For this review, take the finished solid that the model builds, in its own axes (mm). Face numbers are marked on the shaded views. A direction names the side the tool comes from. Round coordinates to 2 decimals unless told otherwise and drop trailing zeros. Order: outer loops, then holes, each group sorted by start corner. A loop starts at its lowest first (then second) coordinate and runs counter-clockwise, first axis right, second up. Notation, with made-up numbers: (26, 69.25) -> (58, 69.25) arc R33 ccw to (58, 98.25) -> close; hole circle Ø2 at (-14, 60.25). An arc over 180 degrees is marked (long way). Use a Markdown table: item, result. Add a question column.
1) Consider section D-D (y = 3.5). State the section outline as (x, z) points, plus the area to 3 significant figures.
2) Draft analysis for pull direction X (two halves, no side actions). For the marked faces 1, 2, 3 and 4, state which applies: pulls with the +X half, pulls with the -X half, needs draft (parallel to the pull), parting line crosses it, or undercut.
3) Wall thickness on line 1 along Y through (x, z) = (3.5, 1.3); line 2 along X through (y, z) = (2.5, 2.5); line 3 along Z through (x, y) = (54.25, -1): over which ranges is each line inside the solid? List them lowest first. Write a range as [from, to].
4) Clearance check with flat-ended pins moving along their axes: P1, Ø1, axis at x = 86, y = 44.5, coming from the -Z side; P2, Ø12, axis at x = 65.5, y = 27.5, coming from the -Z side; P3, Ø3, axis at x = 56, z = 5.5, coming from the +Y side. State where each tip first meets the part, or that it passes through.
5) Consider section B-B (x = 3.5). State the section outline as (y, z) points.
6) Machinability: for the marked faces 5, 6, 7 and 8, which of the approach directions +Z, -Z, +X, -X, +Y, -Y give a long, thin tool a straight path to every point of the face, cutting with its end or side? Answer none if there is none.
7) Consider section C-C (z = 12.25). State the section outline as (x, y) points.
8) Consider section A-A (y = 52.5). State the section outline as (x, z) points, plus the area to 3 significant figures.
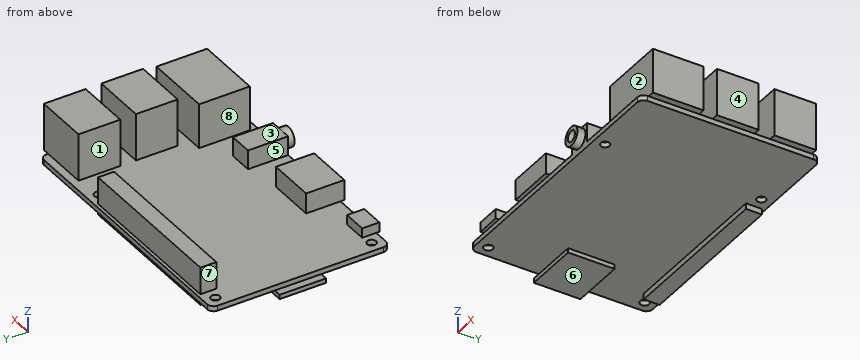
```python
from build123d import *

# Parameters (mm, degrees)
F0_R      = 1.4
F1_DEPTH  = 1.6
F2_W      = 15.1
F2_H      = 13.1
F2_W_2    = 2.1
F3_DEPTH  = 14.8
F2_W_3    = 19.1
F2_H_2    = 15.9
F4_DEPTH  = 14
F5_W      = 50.8
F5_H      = 5
F6_DEPTH  = 8.5
F7_DEPTH  = 3.4
F8_W      = 17
F8_H      = 14.6
F9_DEPTH  = 1.4
F10_W     = 7.5
F10_H     = 4.4
F10_H_2   = 1
F11_DEPTH = 3
F10_W_2   = 15
F10_H_3   = 10.8
F10_H_4   = 1.2
F12_DEPTH = 6.4
F10_H_5   = 12.6
F13_DEPTH = 6
F14_R     = 3
F14_R_2   = 1.75
F15_DEPTH = 2.5


with BuildPart() as f1:
    # F0 (on Top) → F1 (new body)
    with BuildSketch(Plane.XY):
        with BuildLine():
            ThreePointArc((0, 2), (0.585786, 0.585786), (2, 0))
            Line((2, 0), (83, 0))
            ThreePointArc((83, 0), (84.414214, 0.585786), (85, 2))
            Line((85, 2), (85, 54))
            ThreePointArc((85, 54), (84.414214, 55.414214), (83, 56))
            Line((83, 56), (2, 56))
            ThreePointArc((2, 56), (0.585786, 55.414214), (0, 54))
            Line((0, 54), (0, 2))
        make_face()
        with Locations((3.5, 3.5)):
            Circle(F0_R, mode=Mode.SUBTRACT)
        with Locations((61.5, 3.5)):
            Circle(F0_R, mode=Mode.SUBTRACT)
        with Locations((3.5, 52.5)):
            Circle(F0_R, mode=Mode.SUBTRACT)
        with Locations((61.5, 52.5)):
            Circle(F0_R, mode=Mode.SUBTRACT)
    extrude(amount=F1_DEPTH)

    # F2 (on face) → F3 (join)
    with BuildSketch(Plane.XY.offset(1.6)):
        with Locations((77.45, 46.95)):
            Rectangle(F2_W, F2_H)
        with Locations((86.05, 46.95)):
            Rectangle(F2_W_2, F2_H)
        with Locations((77.45, 28.95)):
            Rectangle(F2_W, F2_H)
        with Locations((86.05, 28.95)):
            Rectangle(F2_W_2, F2_H)
    extrude(amount=F3_DEPTH)

    # F2 (on face) → F4 (join)
    with BuildSketch(Plane.XY.offset(1.6)):
        with Locations((75.45, 10.25)):
            Rectangle(F2_W_3, F2_H_2)
        with Locations((86.05, 10.25)):
            Rectangle(F2_W_2, F2_H_2)
    extrude(amount=F4_DEPTH)

    # F5 (on face) → F6 (join)
    with BuildSketch(Plane.XY.offset(1.6)):
        with Locations((32.4, 52.5)):
            Rectangle(F5_W, F5_H)
    extrude(amount=F6_DEPTH)

    # F5 (on face) → F7 (join)
    with BuildSketch(Plane.XY.offset(1.6)):
        with Locations((32.4, 52.5)):
            Rectangle(F5_W, F5_H)
    extrude(amount=-F7_DEPTH)

    # F8 (on face) → F9 (join)
    with BuildSketch(Plane(origin=(0, 0, 0), x_dir=(1, 0, 0), z_dir=(0, 0, -1))):
        with Locations((6.1, -28.8)):
            Rectangle(F8_W, F8_H)
    extrude(amount=F9_DEPTH)

    # F10 (on face) → F11 (join)
    with BuildSketch(Plane.XY.offset(1.6)):
        with Locations((10.55, 2.2)):
            Rectangle(F10_W, F10_H)
        with Locations((10.55, -0.5)):
            Rectangle(F10_W, F10_H_2)
    extrude(amount=F11_DEPTH)

    # F10 (on face) → F12 (join)
    with BuildSketch(Plane.XY.offset(1.6)):
        with Locations((32, 5.4)):
            Rectangle(F10_W_2, F10_H_3)
        with Locations((32, -0.6)):
            Rectangle(F10_W_2, F10_H_4)
    extrude(amount=F12_DEPTH)

    # F10 (on face) → F13 (join)
    with BuildSketch(Plane.XY.offset(1.6)):
        with Locations((54.25, 6.3)):
            Rectangle(F10_W, F10_H_5)
    extrude(amount=F13_DEPTH)

    # F14 (on face) → F15 (join)
    with BuildSketch(Plane.XZ):
        with Locations((54.25, 4.6)):
            Circle(F14_R)
        with Locations((54.25, 4.6)):
            Circle(F14_R_2, mode=Mode.SUBTRACT)
    extrude(amount=F15_DEPTH)


solid = f1.part
```
Results list:
| question | item | result |
|---|---|---|
| 1 | outline | (0, 0) -> (2.1, 0) -> (2.1, 1.6) -> (0, 1.6) -> close; (4.9, 0) -> (60.1, 0) -> (60.1, 1.6) -> (58, 1.6) -> (58, 7.6) -> (50.5, 7.6) -> (50.5, 1.6) -> (39.5, 1.6) -> (39.5, 8) -> (24.5, 8) -> (24.5, 1.6) -> (14.3, 1.6) -> (14.3, 4.6) -> (6.8, 4.6) -> (6.8, 1.6) -> (4.9, 1.6) -> close; (62.9, 0) -> (85, 0) -> (85, 1.6) -> (87.1, 1.6) -> (87.1, 15.6) -> (65.9, 15.6) -> (65.9, 1.6) -> (62.9, 1.6) -> close |
| 1 | area | 587 mm2 |
| 2 | face 1 | undercut |
| 2 | face 2 | needs draft |
| 2 | face 3 | undercut |
| 2 | face 4 | pulls with the +X half |
| 3 | line 1 | [0, 2.1], [4.9, 51.1], [53.9, 56] |
| 3 | line 2 | [6.8, 14.3], [24.5, 39.5], [50.5, 58], [65.9, 87.1] |
| 3 | line 3 | [1.6, 2.85], [6.35, 7.6] |
| 4 | P1 | z = 1.6 |
| 4 | P2 | z = 0 |
| 4 | P3 | y = 55 |
| 5 | outline | (0, 0) -> (2.1, 0) -> (2.1, 1.6) -> (0, 1.6) -> close; (4.9, 0) -> (21.5, 0) -> (21.5, -1.4) -> (36.1, -1.4) -> (36.1, 0) -> (51.1, 0) -> (51.1, 1.6) -> (4.9, 1.6) -> close; (53.9, 0) -> (56, 0) -> (56, 1.6) -> (53.9, 1.6) -> close |
| 6 | face 5 | +Z, -Y |
| 6 | face 6 | -Z, +X, -X, -Y |
| 6 | face 7 | +Z, -X, +Y |
| 6 | face 8 | +Z, +Y, -Y |
| 7 | outline | (65.9, 2.3) -> (87.1, 2.3) -> (87.1, 18.2) -> (65.9, 18.2) -> close; (69.9, 22.4) -> (87.1, 22.4) -> (87.1, 35.5) -> (69.9, 35.5) -> close; (69.9, 40.4) -> (87.1, 40.4) -> (87.1, 53.5) -> (69.9, 53.5) -> close |
| 8 | outline | (0, 0) -> (2.1, 0) -> (2.1, 1.6) -> (0, 1.6) -> close; (4.9, 0) -> (7, 0) -> (7, -1.8) -> (57.8, -1.8) -> (57.8, 0) -> (60.1, 0) -> (60.1, 1.6) -> (57.8, 1.6) -> (57.8, 10.1) -> (7, 10.1) -> (7, 1.6) -> (4.9, 1.6) -> close; (62.9, 0) -> (85, 0) -> (85, 1.6) -> (87.1, 1.6) -> (87.1, 16.4) -> (69.9, 16.4) -> (69.9, 1.6) -> (62.9, 1.6) -> close |
| 8 | area | 905 mm2 |
